The figure shows three views and two pictorial views of one solid part (mm, origin at its lowest corner). Answer the questions. A direction names the side the tool comes from. Coordinates: 2 decimals unless noted, no trailing zeros. Order: outer loops, then holes, each group sorted by start corner. A loop starts at its lowest first (then second) coordinate and runs counter-clockwise, first axis right, second up. Notation, with made-up numbers: M -3.75,63.25 L 46.25,63.25 A26 cw 46.25,77.25 Z; hole C 68,44.25 d8. An arc over 180 degrees is marked long. Write item = value, one per line. Start each with the question number.
Q1. Each of these flat-tipped pins is pushed along its axis until it touches: P1, Ø8, axis at y = 24, z = 92.5, coming from the -X side; P2, Ø6, axis at x = 11, y = 9, coming from the -Z side. Where does it stop, or does it pass through?
Q2. Find section B-B on x = 14.5. Give the vertices of the cut face in (y, z), and give its area (3 significant figures).
Q3. A tool of negligible diameter and unlimited length cuts with its end or side. For the marked faces 1 and 2, from which of +Z, -Z, +X, -X, +Y, -Y can it reach the whole face along a straight path? Write none if from no direction.
Q4. Find section C-C on z = 31.5. Give the vertices of the cut face in (x, y), and give its area (3 significant figures).
Q5. Find section A-A on y = 17.5. Give the vertices of the cut face in (x, z).
Q6. Straight lines are drawn through the part: line 1 along X through (y, z) = (3, 54); line 2 along Z through (x, y) = (18, 21). For each, find the intervals that lie inside material, in ascending order.
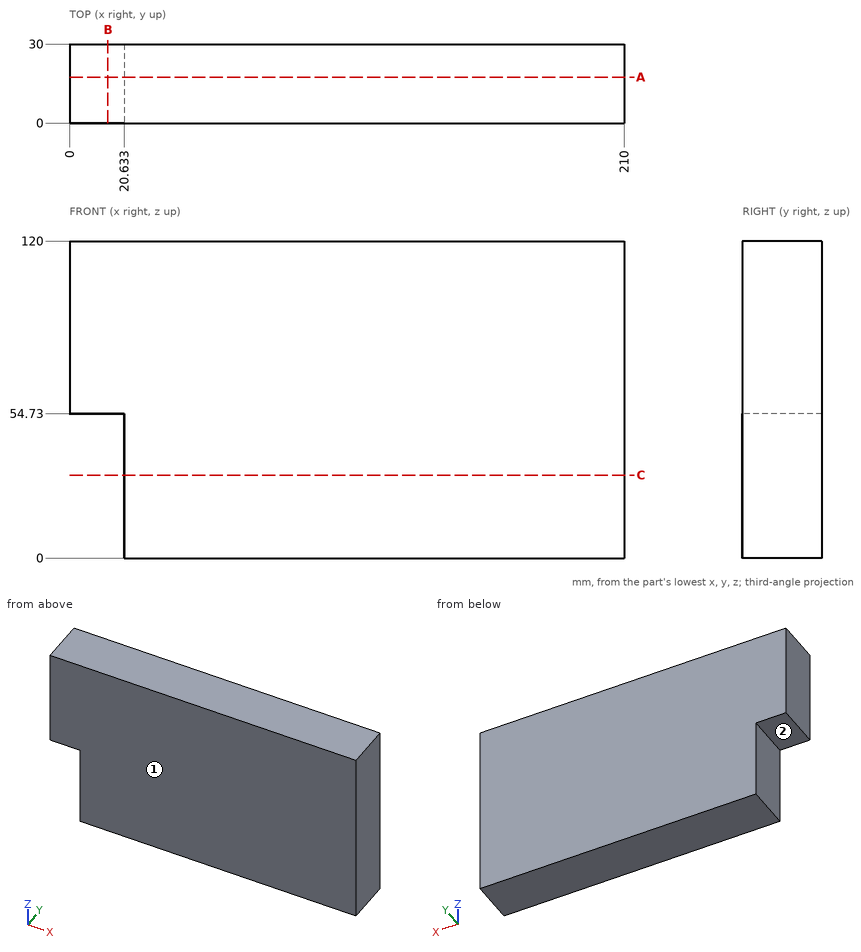
Findings below:
q1.P1 = 0
q1.P2 = 54.73
q2.outline = M 0,54.73 L 30,54.73 L 30,120 L 0,120 Z
q2.area = 1,960 mm^2
q3.face_1 = +Z, -Z, +X, -X, -Y
q3.face_2 = -Z, -X, +Y, -Y
q4.outline = M 20.63,0 L 210,0 L 210,30 L 20.63,30 Z
q4.area = 5,680 mm^2
q5.outline = M 0,54.73 L 20.63,54.73 L 20.63,0 L 210,0 L 210,120 L 0,120 Z
q6.line_1 = 20.63 to 210
q6.line_2 = 54.73 to 120
